```python
from build123d import *

# Parameters (mm, degrees)
SKETCH1_W           = 50
SKETCH1_H           = 50
SKETCH1_W_2         = 47
SKETCH1_H_2         = 47
BOSS_EXTRUDE1_DEPTH = 900
SKETCH2_R           = 2
CUT_EXTRUDE1_DEPTH  = 59
CUT_EXTRUDE2_DEPTH  = 10
CUT_EXTRUDE3_DEPTH  = 10
SKETCH5_R           = 3
CUT_EXTRUDE4_DEPTH  = 55
SKETCH6_R           = 3.125
SKETCH6_R_2         = 5
CUT_EXTRUDE5_DEPTH  = 70


with BuildPart() as part:
    # Sketch1 → Boss-Extrude1 (new body)
    with BuildSketch(Plane.XY):
        Rectangle(SKETCH1_W, SKETCH1_H)
        Rectangle(SKETCH1_W_2, SKETCH1_H_2, mode=Mode.SUBTRACT)
    extrude(amount=BOSS_EXTRUDE1_DEPTH)

    # Sketch2 → Cut-Extrude1 (cut)
    with BuildSketch(Plane(origin=(25, 0, 0), x_dir=(0, 0, -1), z_dir=(1, 0, 0))):
        with Locations((-450, -15)):
            Circle(SKETCH2_R)
        with Locations((-427, 10)):
            Circle(SKETCH2_R)
        with Locations((-473, 10)):
            Circle(SKETCH2_R)
    extrude(amount=-CUT_EXTRUDE1_DEPTH, mode=Mode.SUBTRACT)

    # Sketch3 → Cut-Extrude2 (cut)
    with BuildSketch(Plane(origin=(0, 25, 0), x_dir=(1, 0, 0), z_dir=(0, 1, 0))):
        with BuildLine():
            Line((14, -843), (14, -913.98611775))
            ThreePointArc((14, -913.98611775), (0, -927.98611775), (-14, -913.98611775))
            Line((-14, -913.98611775), (-14, -843))
            ThreePointArc((-14, -843), (0, -829), (14, -843))
        make_face()
    cut_extrude2 = extrude(amount=-CUT_EXTRUDE2_DEPTH, mode=Mode.SUBTRACT)

    # Sketch4 → Cut-Extrude3 (cut)
    with BuildSketch(Plane.XZ.offset(25)):
        with BuildLine():
            Line((-17.498938419, 850), (-17.498938419, 939.078503923))
            ThreePointArc((-17.498938419, 939.078503923), (0.001061581, 956.578503923), (17.501061581, 939.078503923))
            Line((17.501061581, 939.078503923), (17.501061581, 850))
            ThreePointArc((17.501061581, 850), (0.001061581, 832.5), (-17.498938419, 850))
        make_face()
    cut_extrude3 = extrude(amount=-CUT_EXTRUDE3_DEPTH, mode=Mode.SUBTRACT)

    # Sketch5 → Cut-Extrude4 (cut)
    with BuildSketch(Plane(origin=(25, 0, 0), x_dir=(0, 0, -1), z_dir=(1, 0, 0))):
        with Locations((-882.5, 11)):
            Circle(SKETCH5_R)
        with Locations((-882.5, -11)):
            Circle(SKETCH5_R)
        with Locations((-816.5, -11)):
            Circle(SKETCH5_R)
        with Locations((-816.5, 11)):
            Circle(SKETCH5_R)
    cut_extrude4 = extrude(amount=-CUT_EXTRUDE4_DEPTH, mode=Mode.SUBTRACT)

    # Mirror1: Cut-Extrude2, Cut-Extrude3, Cut-Extrude4 across plane
    add(cut_extrude2.mirror(Plane.XY.offset(450)), mode=Mode.SUBTRACT)
    add(cut_extrude3.mirror(Plane.XY.offset(450)), mode=Mode.SUBTRACT)
    add(cut_extrude4.mirror(Plane.XY.offset(450)), mode=Mode.SUBTRACT)

    # Sketch6 → Cut-Extrude5 (cut)
    with BuildSketch(Plane(origin=(0, 25, 0), x_dir=(1, 0, 0), z_dir=(0, 1, 0))):
        with Locations((0, -694.2275)):
            Circle(SKETCH6_R)
        with Locations((0, -739.8525)):
            Circle(SKETCH6_R)
        with Locations((0, -717.04)):
            Circle(SKETCH6_R_2)
    cut_extrude5 = extrude(amount=-CUT_EXTRUDE5_DEPTH, mode=Mode.SUBTRACT)

    # Mirror2: Cut-Extrude5 across plane
    add(cut_extrude5.mirror(Plane.XY.offset(450)), mode=Mode.SUBTRACT)


solid = part.part
```
Work out the finished part from the listing and answer in its coordinate system (mm). A direction names the side the tool comes from. Coordinates: 2 decimals unless noted, no trailing zeros. Order: outer loops, then holes, each group sorted by start corner. A loop starts at its lowest first (then second) coordinate and runs counter-clockwise, first axis right, second up. Notation, with made-up numbers: M -19,-16.5 L 30,-16.5 A8 ccw 30,-3.5 Z; hole C 84,8.25 d7. An arc over 180 degrees is marked long. Use CSV: the item, a comma, the result in double quotes.
1) Determine the mould class of faces 6 (the face through (23.5, 0, 444)), 7 (the face through (0, 24, 71)), 8 (the face through (0, -25, 444)) for opening direction Y: released by +Y, released by -Y, zero draft, split by the parting line, or undercut.
Worked out:
face 6,"undercut"
face 7,"zero draft"
face 8,"released by -Y"
2) Section A-A on z = 241 is taken. Write down the section's boundary in (x, y).
Worked out:
outline,"M -25,-25 L 25,-25 L 25,25 L -25,25 Z; hole M -23.5,-23.5 L 23.5,-23.5 L 23.5,23.5 L -23.5,23.5 Z"
3) Consider line 1 (Y direction, x = 24, z = 882); line 2 (X direction, y = 5.5, z = 235). Determine where each line is inside the solid, lowest interval first. Write a range as [from, to].
Worked out:
line 1,"y = [-25, -13.96], [-8.04, 8.04], [13.96, 25]"
line 2,"x = [-25, -23.5], [23.5, 25]"
4) For faces 1 (the face through (0.386, -24.26, 67.496)), 2 (the face through (0, 24, 829)), 3 (the face through (0.386, -24.26, 832.504)), 4 (the face through (0, 23.5, 444)), 5 (the face through (0, 25, 444)), determine the directions among +Z, -Z, +X, -X, +Y, -Y from which every point of the face is accessible in a straight line to the end or side of a thin tool.
Worked out:
face 1,"-Z, -Y"
face 2,"+Z, +Y"
face 3,"+Z, -Y"
face 4,"+Z, -Z"
face 5,"+Z, -Z, +X, -X, +Y"
